Geometry check sheet. Reference: the model listing, model coordinates, mm. A direction names the side the tool comes from. Give positions to 0.01 mm unless a question says otherwise; leave off trailing zeros. Write each loop counter-clockwise with the first axis right and the second up, starting at its lowest first coordinate (ties: lowest second). Pieces come first, ordered by that corner, then holes. Notation, with made-up numbers: (64, -18.5) -> (108, -18.5) arc R27 cw to (108, 10.5) -> close; hole circle Ø3 at (-22.75, -12.5). An arc over 180 degrees is marked (long way). Write item = value, one per line. Start each with the question number.
1. Cross-section at C-C, the plane z = 1.5. Record the cut outline in (x, y), plus the area to 3 significant figures.
2. Thickness scan on line 1 along X through (y, z) = (0, 1.9); line 2 along X through (y, z) = (14, 1.4); line 3 along Y through (x, z) = (0, 1.1). Record the ranges inside material, lowest first.
3. Depth check by flat-ended pin: P1, Ø5, axis at x = 0, y = 0, coming from the -Z side. Enter the tip coordinate at first touch or a pass-through.
4. Set-up check for faces 1 (the cylindrical face through (-17.424, -33.882, 1.252)), 2 (the flat face through (15.662, 12.547, 1.288)): record each of +Z, -Z, +X, -X, +Y, -Y from which the full face is reachable in a straight line by a thin tool's end or side.
5. Cross-section at A-A, the plane y = 0. Record the cut outline in (x, z), plus the area to 3 significant figures.
6. Cross-section at B-B, the plane x = -28. Record the cut outline in (y, z).
```python
from build123d import *

# Parameters (mm, degrees)
SKETCH1_R           = 38.1
BOSS_EXTRUDE1_DEPTH = 2.54
CUT_EXTRUDE1_DEPTH  = 2.54
SKETCH3_R           = 1.524
CUT_EXTRUDE2_DEPTH  = 2.54


with BuildPart() as part:
    # Sketch1 → Boss-Extrude1 (new body)
    with BuildSketch(Plane.XY):
        Circle(SKETCH1_R)
    extrude(amount=BOSS_EXTRUDE1_DEPTH)

    # Sketch2 → Cut-Extrude1 (cut)
    with BuildSketch(Plane.XY.offset(2.54)):
        with BuildLine():
            Line((0, 0), (-0.783784717, 38.091937225))
            ThreePointArc((-0.783784717, 38.091937225), (16.139227372, 34.512828627), (29.735705264, 23.820114031))
            Line((29.735705264, 23.820114031), (0, 0))
        make_face()
    extrude(amount=-CUT_EXTRUDE1_DEPTH, mode=Mode.SUBTRACT)

    # Sketch3 → Cut-Extrude2 (cut)
    with BuildSketch(Plane.XY.offset(2.54)):
        Circle(SKETCH3_R)
    extrude(amount=-CUT_EXTRUDE2_DEPTH, mode=Mode.SUBTRACT)


solid = part.part
```
Answers:
q1.outline = (-0.78, 38.09) arc R38.1 ccw (long way) to (29.74, 23.82) -> (1.19, 0.95) arc R1.52 cw (long way) to (-0.03, 1.52) -> close
q1.area = 3,890 mm^2
q2.line_1 = -38.1 to -1.52, 1.52 to 38.1
q2.line_2 = -35.43 to -0.29, 17.48 to 35.43
q2.line_3 = -38.1 to -1.52
q3.P1 = 0
q4.face_1 = +Z, -Z
q4.face_2 = +Z, -Z, +Y
q5.outline = (-38.1, 0) -> (-1.52, 0) -> (-1.52, 2.54) -> (-38.1, 2.54) -> close; (1.52, 0) -> (38.1, 0) -> (38.1, 2.54) -> (1.52, 2.54) -> close
q5.area = 186 mm^2
q6.outline = (-25.84, 0) -> (25.84, 0) -> (25.84, 2.54) -> (-25.84, 2.54) -> close
